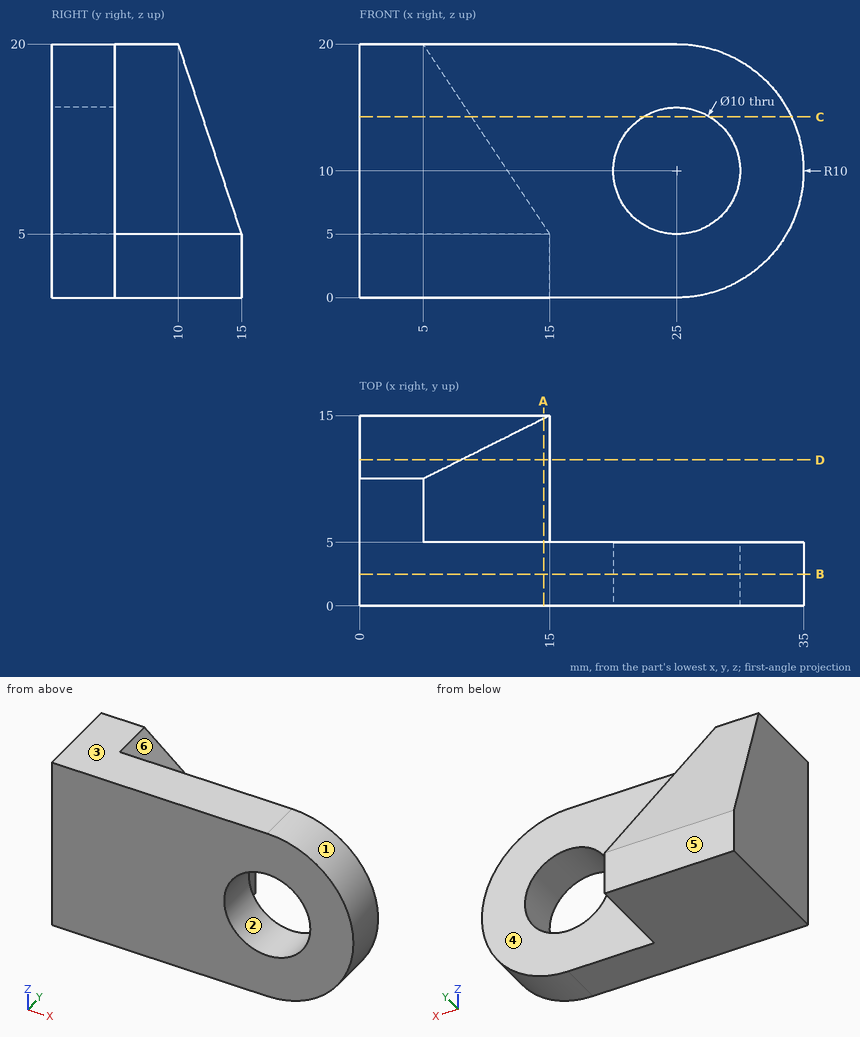
Could you check a few things on this drawing? It's one solid part, dimensions in mm from its lowest x, y, z. A direction names the side the tool comes from. Coordinates: 2 decimals unless noted, no trailing zeros. Loops run counter-clockwise (first coordinate to the right, second up) from the corner with the lowest first, then second, coordinate; pieces in that order, holes last. Notation, with made-up numbers: (64.5, 51.5) - (110.5, 51.5) arc R18 ccw to (110.5, 62.5) - close; hole circle Ø6 at (-11.75, -36). An arc over 180 degrees is marked (long way). Return JSON: item names as keys, results as strings. Group by question number.
Item 1: Will these pins go through, and if not, where does the flat tip stop? P1, Ø4, axis at x = 25, z = 15.5, coming from the +Y side; P2, Ø4, axis at y = 10.5, z = 2, coming from the +X side; P3, Ø5, axis at x = 12.5, y = 8, coming from the +Z side.
Item 2: On a 3-axis mill with a long thin cutter (end or side, diameter ignored), from which of +Z, -Z, +X, -X, +Y, -Y can I reach the whole of each face in a straight line? I mean the marked faces 5 and 6. Say none if no direction works.
Item 3: If we section it at C-C on z = 14.25: Write out the boundary of the cut face in (x, y).
Item 4: We'd pull the mould along Z, two halves only. Please class the marked faces 1, 2, 3 and 4: +Z half, -Z half, draft (parallel to the pull), parting line (faces both ways), or undercut.
Item 5: If we section it at A-A on x = 14.5: Write out the boundary of the cut face in (y, z), and give its area (3 significant figures).
Item 6: If we section it at D-D on y = 11.5: Write out the boundary of the cut face in (x, z), and give its area (3 significant figures).
Item 7: If we section it at B-B on y = 2.5: Write out the boundary of the cut face in (x, z).
Item 8: I need wall thicknesses on line 1 (X direction, y = 2.35, z = 10); line 2 (Z direction, x = 25, y = 2.75); line 3 (Y direction, x = 18.5, z = 8.25). Which ranges of each line are inside material? Lowest first, please. Write a range as from..to.
Calculated:
{
 "1": {"P1": "stops at y = 5", "P2": "stops at x = 15", "P3": "stops at z = 12.5"},
 "2": {"face 5": "+Z, -Z, +X, -X, +Y", "face 6": "+Z, +X, +Y"},
 "3": {"outline": "(0, 0) - (22.37, 0) - (22.37, 5) - (8.83, 5) - (8.83, 11.92) - (0, 11.92) - close; (27.63, 0) - (34.05, 0) - (34.05, 5) - (27.63, 5) - close"},
 "4": {"face 1": "parting line", "face 2": "undercut", "face 3": "+Z half", "face 4": "draft"},
 "5": {"outline": "(0, 0) - (15, 0) - (15, 5) - (14.75, 5.75) - (5, 5.75) - (5, 20) - (0, 20) - close", "area": "157 mm^2"},
 "6": {"outline": "(0, 0) - (15, 0) - (15, 5) - (8, 15.5) - (0, 15.5) - close", "area": "196 mm^2"},
 "7": {"outline": "(0, 0) - (25, 0) arc R10 ccw to (25, 20) - (0, 20) - close; hole circle Ø10 at (25, 10)"},
 "8": {"line 1": "x = 0..20, 30..35", "line 2": "z = 0..5, 15..20", "line 3": "y = 0..5"}
}
